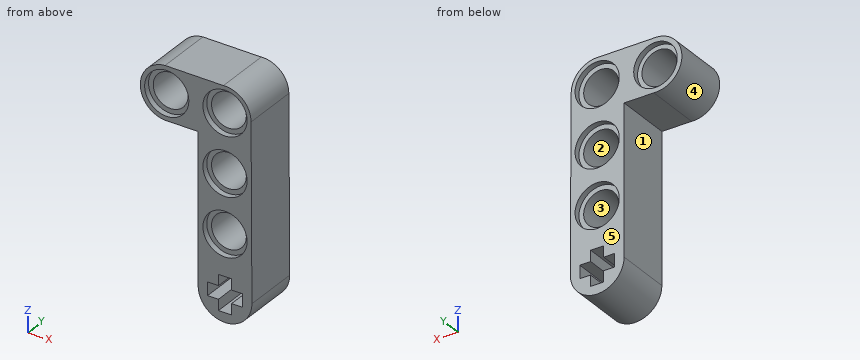
```python
from build123d import *

# Parameters (mm, degrees)
SKETCH1_R           = 2.4
BOSS_EXTRUDE2_DEPTH = 7.8
SKETCH2_R           = 3.005
SKETCH2_R_2         = 3.05
CUT_EXTRUDE1_DEPTH  = 0.8
SKETCH3_R           = 3.05
CUT_EXTRUDE2_DEPTH  = 0.8


with BuildPart() as part:
    # Sketch1 → Boss-Extrude2 (new body)
    with BuildSketch(Plane(origin=(0, 0, 0), x_dir=(1, 0, 0), z_dir=(0, 1, 0))):
        with BuildLine():
            Line((-3.723198341, 3.643010683), (0.380925068, 3.643010683))
            Line((0.380925068, 3.643010683), (0.380925068, 24.12))
            ThreePointArc((0.380925068, 24.12), (4.090929192, 27.830004128), (7.800933325, 24.120000008))
            Line((7.800933325, 24.120000008), (7.680923984, 0.007228348))
            ThreePointArc((7.680923984, 0.007228348), (6.551552066, -2.614086822), (3.866782865, -3.582997801))
            Line((3.866782865, -3.582997801), (-4.174942755, -3.643002442))
            ThreePointArc((-4.174942755, -3.643002442), (-7.592081486, 0.225872463), (-3.723198341, 3.643010683))
        make_face()
        with Locations((-3.949070804, 0)):
            Circle(SKETCH1_R, mode=Mode.SUBTRACT)
        with Locations((4.090929196, 0)):
            Circle(SKETCH1_R, mode=Mode.SUBTRACT)
        with Locations((4.090929196, 8.04)):
            Circle(SKETCH1_R, mode=Mode.SUBTRACT)
        with Locations((4.090929196, 16.08)):
            Circle(SKETCH1_R, mode=Mode.SUBTRACT)
        Polygon((3.190929196, 26.52), (4.990929196, 26.52), (4.990929196, 25.02), (6.490929196, 25.02), (6.490929196, 23.22), (4.990929196, 23.22), (4.990929196, 21.72), (3.190929196, 21.72), (3.190929196, 23.22), (1.690929196, 23.22), (1.690929196, 25.02), (3.190929196, 25.02), align=None, mode=Mode.SUBTRACT)
    extrude(amount=BOSS_EXTRUDE2_DEPTH)

    # Sketch2 → Cut-Extrude1 (cut)
    with BuildSketch(Plane(origin=(0, 7.8, 0), x_dir=(1, 0, 0), z_dir=(0, 1, 0))):
        with Locations((-3.949070804, 0)):
            Circle(SKETCH2_R)
        with Locations((4.090929196, 0)):
            Circle(SKETCH2_R_2)
        with Locations((4.090929196, 8.04)):
            Circle(SKETCH2_R_2)
        with Locations((4.090929196, 16.08)):
            Circle(SKETCH2_R_2)
    extrude(amount=-CUT_EXTRUDE1_DEPTH, mode=Mode.SUBTRACT)

    # Sketch3 → Cut-Extrude2 (cut)
    with BuildSketch(Plane.XZ):
        with Locations((-3.949070804, 0)):
            Circle(SKETCH3_R)
        with Locations((4.090929196, 0)):
            Circle(SKETCH3_R)
        with Locations((4.090929196, -8.04)):
            Circle(SKETCH3_R)
        with Locations((4.090929196, -16.08)):
            Circle(SKETCH3_R)
    extrude(amount=-CUT_EXTRUDE2_DEPTH, mode=Mode.SUBTRACT)


solid = part.part
```
Check sheet for the modelled part. Datum: model origin and axes. Units: mm. Face numbers are marked on the shaded views. A direction names the side the tool comes from. Coordinates: 2 decimals unless noted, no trailing zeros. Write each loop counter-clockwise with the first axis right and the second up, starting at its lowest first coordinate (ties: lowest second). Pieces come first, ordered by that corner, then holes. Notation, with made-up numbers: M 20,-20.75 L 76,-20.75 A31 ccw 76,5.25 Z; hole C 56,-14.75 d7. An arc over 180 degrees is marked long. Use one line per item in the form item = value.
Item 1: Material ranges on L1, parallel to Z at x = 4, y = 1.5; L2, parallel to Z at x = 4, y = 7.25; L3, parallel to X at y = 7.25, z = 0, recorded low to high. Write a range as from..to.
Answer below:
L1 = -27.83..-26.52, -21.72..-18.48, -13.68..-10.44, -5.64..-2.4, 2.4..3.59
L2 = -27.83..-26.52, -21.72..-19.13, -13.03..-11.09, -4.99..-3.05, 3.05..3.59
L3 = -7.6..-6.95, -0.94..1.04, 7.14..7.68
Item 2: Sectioned sample at C-C, the plane z = -16.08. Record the cut outline in (x, y), and give its area (3 significant figures).
Answer below:
outline = M 0.38,0 L 1.04,0 L 1.04,0.8 L 1.69,0.8 L 1.69,7 L 1.04,7 L 1.04,7.8 L 0.38,7.8 Z; M 6.49,0.8 L 7.14,0.8 L 7.14,0 L 7.76,0 L 7.76,7.8 L 7.14,7.8 L 7.14,7 L 6.49,7 Z
area = 18.0 mm^2
Item 3: Sectioned sample at A-A, the plane y = 6.25. Record the cut outline in (x, z).
Answer below:
outline = M -4.17,3.64 A3.65 ccw -3.72,-3.64 L 0.38,-3.64 L 0.38,-24.12 A3.71 ccw 7.8,-24.12 L 7.68,-0.01 A3.59 ccw 3.87,3.58 Z; hole C -3.95,0 d4.8; hole M 1.69,-25.02 L 3.19,-25.02 L 3.19,-26.52 L 4.99,-26.52 L 4.99,-25.02 L 6.49,-25.02 L 6.49,-23.22 L 4.99,-23.22 L 4.99,-21.72 L 3.19,-21.72 L 3.19,-23.22 L 1.69,-23.22 Z; hole C 4.09,-16.08 d4.8; hole C 4.09,-8.04 d4.8; hole C 4.09,0 d4.8
Item 4: Set-up check for the marked faces 1 and 2: record each of +Z, -Z, +X, -X, +Y, -Y from which the full face is reachable in a straight line by a thin tool's end or side.
Answer below:
face_1 = -Z, -X, +Y, -Y
face_2 = +Y, -Y
Item 5: Sectioned sample at B-B, the plane x = -2. Record the cut outline in (y, z), and give its area (3 significant figures).
Answer below:
outline = M 0,-3.64 L 7.8,-3.64 L 7.8,-2.29 L 7,-2.29 L 7,-1.4 L 0.8,-1.4 L 0.8,-2.35 L 0,-2.35 Z; M 0,2.35 L 0.8,2.35 L 0.8,1.4 L 7,1.4 L 7,2.29 L 7.8,2.29 L 7.8,3.63 L 0,3.63 Z
area = 31.9 mm^2
Item 6: Release check for a two-part mould opening along Z. For the marked faces 3, 4 and 5 record: pulls with the +Z half, pulls with the -Z half, needs draft (parallel to the pull), parting line crosses it, or undercut.
Answer below:
face_3 = undercut
face_4 = parting line crosses it
face_5 = needs draft
Item 7: Gauge pin test, flat ends, axial feed: pin 1 Ø1.5 at (x, y) = (5, 2) entering from -Z; pin 2 Ø5 at (x, z) = (4.09, -16.08) entering from -Y; pin 3 Ø3.5 at (x, y) = (-0.5, 2.5) entering from -Z. Record the tip position at first contact, or that the pin passes through.
Answer below:
pin_1 = -27.83
pin_2 = 0.8
pin_3 = -26.51
